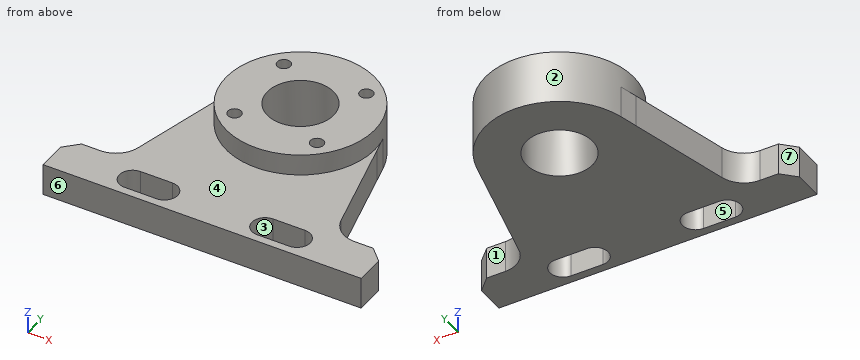
Autodesk Inventor part; units mm, degrees
ref_plane "YZ Plane" through (0, 0, 0) normal (1, 0, 0) x (0, 1, 0)
ref_plane "XZ Plane" through (0, 0, 0) normal (0, 1, 0) x (-1, 0, 0)
ref_plane "XY Plane" through (0, 0, 0) normal (0, 0, 1) x (1, 0, 0)
sketch "스케치1" plane through (0, 0, 0) normal (0, 0, 1) x (1, 0, 0)
  line L0 (-60, 0) -> (60, 0)
  line L1 (60, 0) -> (60, 62)
  line L2 (-60, 62) -> (-60, 0)
  line L3 (0, 0) -> (0, 151.2751)
  arc A0 (-31, 13) -> (-31, 3) centre (-31, 8) ccw
  arc A1 (-19, 3) -> (-19, 13) centre (-19, 8) ccw
  line L4 (-31, 13) -> (-19, 13)
  line L5 (-31, 3) -> (-19, 3)
  arc A2 (31, 3) -> (31, 13) centre (31, 8) ccw
  arc A3 (19, 13) -> (19, 3) centre (19, 8) ccw
  line L6 (31, 13) -> (19, 13)
  line L7 (31, 3) -> (19, 3)
  arc A4 (28, 62) -> (-28, 62) centre (0, 62) ccw
  line L8 (60, 62) -> (28, 62)
  line L9 (-28, 62) -> (-60, 62)
  dimension "d0" = 120
  dimension "d1" = 62
  dimension "d2" = 29
  dimension "d3" = 10
  dimension "d5" = 10
  dimension "d6" = 12
  dimension "d7" = 56
  dimension "d8" = 8
extrude "돌출1" add sketch "스케치1" along normal blind 12
sketch "스케치2" plane through (0, 0, 12) normal (0, 0, 1) x (1, 0, 0)
  circle A0 centre (0, 62) radius 28
  arc A1 (28, 62) -> (-28, 62) centre (0, 62) ccw
  point P0 (0, 0)
  dimension "d11" = 56
extrude "돌출2" add sketch "스케치2" along normal blind 8
sketch "스케치3" plane through (0, 0, 12) normal (0, 0, 1) x (1, 0, 0)
  arc A0 (-48, 16) -> (-48, 36) centre (-48, 26) ccw
  line L0 (-48, 16) -> (-80.7935, 16)
  line L1 (-80.7935, 16) -> (-80.7935, 63.6006)
  line L2 (-80.7935, 63.6006) -> (-48, 63.6006)
  line L3 (-48, 63.6006) -> (-48, 36)
  line L4 (-60, 0) -> (60, 0)
  line L5 (-60, 62) -> (-60, 0)
  point P0 (0, 0)
  dimension "d14" = 20
  dimension "d15" = 16
  dimension "d16" = 12
extrude "돌출3" cut sketch "스케치3" against normal blind 20
mirror "미러1" about plane through (0, 0, 0) normal (1, 0, 0) of "돌출3"
chamfer "모따기1" distance 5 angle 45 2 edges at (-60, 16, 6) (60, 16, 6)
sketch "스케치4" plane through (0, 0, 12) normal (0, 0, 1) x (1, 0, 0)
  line L0 (-38.2901, 23.609) -> (-27.1878, 68.6949)
  circle A0 centre (0, 62) radius 28
  arc A1 (-48, 16) -> (-48, 36) centre (-48, 26) ccw
  line L1 (0, 0) -> (0, 106.1688)
  line L2 (27.1878, 68.6949) -> (38.2901, 23.609)
  arc A2 (48, 36) -> (48, 16) centre (48, 26) ccw
  line L3 (-48, 16) -> (-74.8883, 57.476)
  line L4 (-74.8883, 57.476) -> (-15.255, 104.9361)
  line L5 (-15.255, 104.9361) -> (38.38, 97.6952)
  line L6 (38.38, 97.6952) -> (82.1306, 43.6078)
  line L7 (82.1306, 43.6078) -> (48, 16)
extrude "돌출4" cut sketch "스케치4" against normal blind 20 contours A1 L3 L4 L5 L1 A0 L0 | L1 L5 L6 L7 A2 L2 A0
sketch "스케치5" plane through (0, 0, 12) normal (0, 0, 1) x (1, 0, 0)
  line L0 (-38.2901, 23.609) -> (-28.8364, 62)
  line L1 (28.8364, 62) -> (28, 62)
  line L2 (28.8364, 62) -> (27.1878, 68.6949)
  line L3 (-27.1878, 68.6949) -> (-28.8364, 62)
  circle A0 centre (0, 62) radius 28
  line L4 (-28.8364, 62) -> (-28, 62)
  line L5 (28, 62) -> (28.8364, 62)
  point P0 (0, 0)
extrude "돌출5" add sketch "스케치5" against normal blind 12 contours L1 A0 L2 | L4 L3 A0
sketch "스케치6" plane through (0, 62, 20) normal (0, 0, 1) x (1, 0, 0)
  circle A0 centre (0, 0) radius 12.5
  circle A1 centre (0, 0) radius 22
  circle A2 centre (15.5563, 15.5563) radius 2.5
  line L0 (-28.2851, -28.2851) -> (32.9008, 32.9008)
  line L1 (-49.5291, 0) -> (47.7327, 0)
  circle A3 centre (0, 0) radius 28
  circle A4 centre (-15.5563, 15.5563) radius 2.5
  circle A5 centre (-15.5563, -15.5563) radius 2.5
  circle A6 centre (15.5563, -15.5563) radius 2.5
  point P0 (0, -62)
  dimension "d29" = 44
  dimension "d26" = 45
  dimension "d27" = 5
  dimension "d28" = 25
  dimension "d32" = 360
extrude "돌출6" cut sketch "스케치6" against normal blind 20 contours L1 L0 A0 | A0 L0 L1 | L0 L1 A0 | A0 L1 L0
extrude "돌출7" cut sketch "스케치6" against normal blind 10 contours L0 A1 A2 | A2 A1 L0 | A5 A1 L0 | L0 A1 A5 | A1 L0 A2 | A6 A1 | A1 A6 | A2 L0 A1 | L0 A5 A1 | A1 A5 L0 | A4 A1 | A1 A4
sketch "스케치7" plane through (0, 62, 20) normal (0, 0, 1) x (1, 0, 0)
  circle A0 centre (15.5563, -15.5563) radius 2.5
  circle A1 centre (0, 0) radius 22
  line L0 (0, -76.267) -> (0, 43.2176)
  point P0 (0, -62)
properties part number "아이들러 풀리 브라켓"
Input: part model. Units: mm. Frame: model coordinates. Face numbers are marked on the shaded views. A direction names the side the tool comes from. Coordinates: 2 decimals unless noted, no trailing zeros. Order: outer loops, then holes, each group sorted by start corner. A loop starts at its lowest first (then second) coordinate and runs counter-clockwise, first axis right, second up.
1. Cut plane D-D, the plane x = 25. Return loops of the section in (y, z).
Checked values:
outline: (0, 0) - (3, 0) - (3, 12) - (0, 12) - close; (13, 0) - (74.61, 0) - (74.61, 20) - (49.39, 20) - (49.39, 12) - (13, 12) - close
2. Access query for the marked faces 1, 2, 3 and 4. Directions: +Z, -Z, +X, -X, +Y, -Y. A direction counts if a zero-diameter tool reaches every point of the face in a straight line with its end or side. Return the directions, or none.
Checked values:
face 1: +Z, -Z, +X, +Y
face 2: +Z
face 3: +Z, -Z
face 4: +Z, -Y
3. Draft query along Y for the marked faces 5, 6 and 7. Return one class per face: +Y half, -Y half, draft (parallel to the pull), parting line (faces both ways), or undercut.
Checked values:
face 5: undercut
face 6: -Y half
face 7: +Y half
4. Ray query, line 1 along X through (y, z) = (44.5, 13.5); line 2 along Y through (x, z) = (0, 7.75); line 3 along Y through (x, z) = (5, 17.5). Return the intervals inside material, ascending.
Checked values:
line 1: x = -21.86 to -17.13, -13.98 to 13.98, 17.13 to 21.86
line 2: y = 0 to 49.5, 74.5 to 90
line 3: y = 34.45 to 50.54, 73.46 to 89.55
5. Cut plane B-B, the plane y = 8. Return loops of the section in (x, z).
Checked values:
outline: (-60, 0) - (-36, 0) - (-36, 12) - (-60, 12) - close; (-14, 0) - (14, 0) - (14, 12) - (-14, 12) - close; (36, 0) - (60, 0) - (60, 12) - (36, 12) - close
6. Cut plane A-A, the plane x = 0. Return loops of the section in (y, z), plus the area to 3 significant figures.
Checked values:
outline: (0, 0) - (49.5, 0) - (49.5, 20) - (34, 20) - (34, 12) - (0, 12) - close; (74.5, 0) - (90, 0) - (90, 20) - (74.5, 20) - close
area: 1,030 mm2
7. Cut plane C-C, the plane z = 2. Return loops of the section in (x, y).
Checked values:
outline: (-60, 0) - (60, 0) - (60, 11) - (55, 16) - (48, 16) arc R10 cw to (38.29, 23.61) - (28.84, 62) - (27.19, 68.69) arc R28 ccw to (-27.19, 68.69) - (-28.84, 62) - (-38.29, 23.61) arc R10 cw to (-48, 16) - (-55, 16) - (-60, 11) - close; hole (-31, 3) - (-19, 3) arc R5 ccw to (-19, 13) - (-31, 13) arc R5 ccw to start; hole circle Ø25 at (0, 62); hole (19, 3) - (31, 3) arc R5 ccw to (31, 13) - (19, 13) arc R5 ccw to start
8. Contact query for flat-ended pins moving along their axis: P1, Ø6, axis at x = -2.5, z = 12.5, coming from the -Y side; P2, Ø2.5, axis at x = 16.5, y = 77, coming from the +Z side; P3, Ø2, axis at x = 50, z = 7, coming from the +Y side; P4, Ø6, axis at x = 23, z = 6, coming from the +Y side. Output: stop coordinate, or through.
Checked values:
P1: stops at y = 0
P2: stops at z = 10
P3: stops at y = 16
P4: stops at y = 81.6
